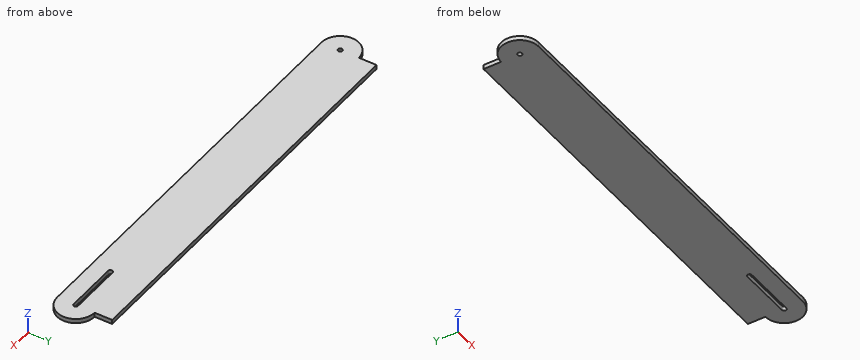
from build123d import *

# Parameters (mm, degrees)
SKETCH1_W           = 584.2
SKETCH1_H           = 25.4
BOSS_EXTRUDE1_DEPTH = 3.175
SKETCH2_R           = 3.175
CUT_EXTRUDE1_DEPTH  = 614.461435473


with BuildPart() as part:
    # Sketch1 → Boss-Extrude1 (new, symmetric)
    with BuildSketch(Plane.XY):
        with Locations((292.1, 39.6875)):
            Rectangle(SKETCH1_W, SKETCH1_H)
        with BuildLine():
            Line((0, -26.9875), (584.2, -26.9875))
            ThreePointArc((584.2, -26.9875), (611.1875, 0), (584.2, 26.9875))
            Line((584.2, 26.9875), (0, 26.9875))
            ThreePointArc((0, 26.9875), (-26.9875, 0), (0, -26.9875))
        make_face()
    extrude(amount=BOSS_EXTRUDE1_DEPTH, both=True)

    # Sketch2 → Cut-Extrude1 (cut, through all)
    with BuildSketch(Plane.XY.offset(3.175)):
        Circle(SKETCH2_R)
        with BuildLine():
            Line((508, 3.175), (584.2, 3.175))
            ThreePointArc((584.2, 3.175), (587.375, 0), (584.2, -3.175))
            Line((584.2, -3.175), (508, -3.175))
            ThreePointArc((508, -3.175), (504.825, 0), (508, 3.175))
        make_face()
    extrude(amount=-CUT_EXTRUDE1_DEPTH, mode=Mode.SUBTRACT)


solid = part.part
Can you work these out from the model? Positions are in its coordinate system, mm. Coordinates: 2 decimals unless noted, no trailing zeros. Order: outer loops, then holes, each group sorted by start corner. A loop starts at its lowest first (then second) coordinate and runs counter-clockwise, first axis right, second up. Notation, with made-up numbers: M -4,78 L 26,78 A31 cw 26,103 Z; hole C 32,-7.75 d5. An arc over 180 degrees is marked long. Answer as CSV lines item,"result".
(1) Suppose I cut it at B-B on z = 1. Count the separate pieces of the cut face and the enclosed holes in it, plus the area to 3 significant figures.
Geometry check:
separate pieces,"1"
enclosed holes,"2"
area,"48,100 mm^2"
(2) Suppose I cut it at A-A on x = 571. Please give me the cut outline in (y, z) (1 decimal), plus the area to 3 significant figures.
Geometry check:
outline,"M -27,-3.2 L -3.2,-3.2 L -3.2,3.2 L -27,3.2 Z; M 3.2,-3.2 L 52.4,-3.2 L 52.4,3.2 L 3.2,3.2 Z"
area,"464 mm^2"
(3) Please list where these lines run through material, in increasing order: L1, parallel to Y at x = 580, z = -2.25 (1 decimal); L2, parallel to X at y = 34, z = 0; L3, parallel to X at y = 11.5, z = -0.75.
Geometry check:
L1,"-27 to -3.2, 3.2 to 52.4"
L2,"0 to 584.2"
L3,"-24.41 to 608.61"
